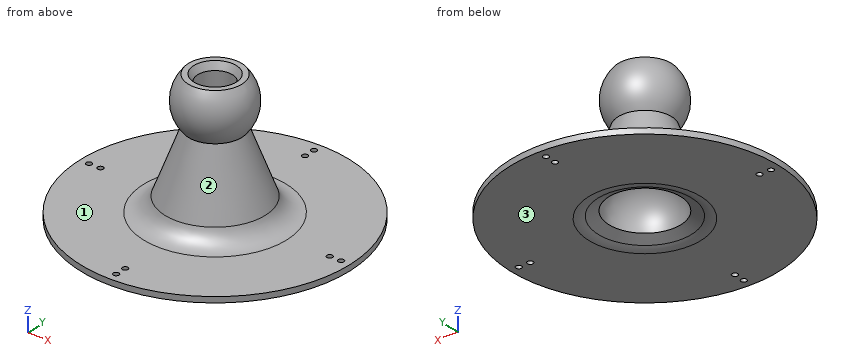
```python
from build123d import *

# Parameters (mm, degrees)
SKETCH2_R          = 28.533493352
CUT_EXTRUDE1_DEPTH = 3.900597164
CUT_EXTRUDE1_DRAFT = -65.378461827
HOLE1_D            = 3.175
HOLE1_DEPTH        = 72.381695866
CHAMFER1_SIZE      = 2.199704526
CHAMFER1_SIZE2     = 3.81
FILLET1_R          = 12.7


with BuildPart() as part:
    # Sketch1 → Revolve1 (revolve)
    with BuildSketch(Plane(origin=(0, 0, 0), x_dir=(1, 0, 0), z_dir=(0, 1, 0))):
        with BuildLine():
            Line((75, 1.293744634), (0, 1.293744634))
            Line((0, 1.293744634), (0, -2.606852529))
            Line((0, -2.606852529), (20.022304736, -2.606852529))
            ThreePointArc((20.022304736, -2.606852529), (17.926393777, -14.259573819), (9.652, -22.727936343))
            Line((9.652, -22.727936343), (9.652, -71.087951232))
            Line((9.652, -71.087951232), (14.88071719, -71.087951232))
            ThreePointArc((14.88071719, -71.087951232), (19.97075, -57.768975616), (14.88071719, -44.45))
            Line((14.88071719, -44.45), (31.064900574, -1.881255366))
            Line((31.064900574, -1.881255366), (75, -1.881255366))
            Line((75, -1.881255366), (75, 1.293744634))
        make_face()
    revolve(axis=Axis((0, 0, -1.293744634), (0, 0, 1)))


with BuildPart() as cut_extrude1_tool:
    # Sketch2 → Cut-Extrude1 (with draft: the straight prism first)
    with BuildSketch(Plane(origin=(0, 0, -1.293744634), x_dir=(-1, 0, 0), z_dir=(0, 0, -1))):
        Circle(SKETCH2_R)
    extrude(amount=-CUT_EXTRUDE1_DEPTH)
    # Cut-Extrude1: the draft: its side faces are tilted about the plane it starts from
    cut_extrude1_sides = [cut_extrude1_tool.faces().sort_by_distance(p)[0] for p in [
        (28.533493352, 0, 0.656553947),
    ]]
    draft(cut_extrude1_sides, Plane(origin=(0, 0, -1.293744634), x_dir=(-1, 0, 0), z_dir=(0, 0, -1)), CUT_EXTRUDE1_DRAFT)


with BuildPart() as part_1:
    add(part.part)

    # Cut-Extrude1: cut by cut_extrude1_tool
    add(cut_extrude1_tool.part, mode=Mode.SUBTRACT)

    # Hole1
    with Locations(Plane(origin=(0, 0, -1.293744634), x_dir=(-1, 0, 0), z_dir=(0, 0, -1))):
        with Locations((-63.5, 0), (-69.85, 0), (0, 63.5), (0, 69.85), (63.5, 0), (69.85, 0), (0, -63.5), (0, -69.85)):
            Hole(HOLE1_D / 2, depth=HOLE1_DEPTH)

    # Chamfer1
    chamfer1_edges = [part_1.edges().sort_by_distance(p)[0] for p in [
        (-9.652, 0, 71.087951232),
    ]]
    chamfer1_side = [part_1.faces().sort_by_distance(p)[0] for p in [
        (-10.072890241, 0, 71.087951232),
    ]]
    chamfer(chamfer1_edges, length=CHAMFER1_SIZE, length2=CHAMFER1_SIZE2, reference=chamfer1_side[0])

    # Fillet1
    fillet1_edges = [part_1.edges().sort_by_distance(p)[0] for p in [
        (-31.064900574, 0, 1.881255366),
        (28.533493352, 0, -1.293744634),
    ]]
    fillet(fillet1_edges, radius=FILLET1_R)


solid = part_1.part
```
The model under review builds one solid part; all positions refer to its coordinate system, in mm. Face numbers are marked on the shaded views. Round coordinates to 2 decimals unless told otherwise and drop trailing zeros. Order: outer loops, then holes, each group sorted by start corner. A loop starts at its lowest first (then second) coordinate and runs counter-clockwise, first axis right, second up. Notation, with made-up numbers: (2.5, -34.75) -> (25.5, -34.75) arc R11 ccw to (25.5, -17.75) -> close; hole circle Ø10 at (-39.75, 49.5). An arc over 180 degrees is marked (long way). Use a Markdown table: item, result.
Q1. Mouldability with a two-part tool opening along Z and no side actions: class the marked faces 1, 2 and 3 as +Z half, -Z half, draft (parallel to the pull), parting line (faces both ways), or undercut.
Values:
| item | result |
|---|---|
| face 1 | +Z half |
| face 2 | undercut |
| face 3 | -Z half |
Q2. We need section A-A on z = 33.5. Write out the cut boundary in (x, y), then the cut area to 3 significant figures.
Values:
| item | result |
|---|---|
| outline | circle Ø38.09 at (0, 0); hole circle Ø19.3 at (0, 0) |
| area | 847 mm^2 |
Q3. We need section B-B on x = 47. Write out the cut boundary in (y, z), then the cut area to 3 significant figures.
Values:
| item | result |
|---|---|
| outline | (-58.45, -1.29) -> (58.45, -1.29) -> (58.45, 1.88) -> (-58.45, 1.88) -> close |
| area | 371 mm^2 |
Q4. Clearance check with flat-ended pins moving along their axes: P1, Ø2.5, axis at x = 63.5, y = 0, coming from the +Z side; P2, Ø1, axis at x = -20, y = -15.5, coming from the -Z side; P3, Ø10, axis at x = 6.5, y = 20.5, coming from the -Z side; P4, Ø8, axis at x = -38, y = -50, coming from the +Z side. State where each tip first meets the part, or that it passes through.
Values:
| item | result |
|---|---|
| P1 | passes through |
| P2 | stops at z = -0.04 |
| P3 | stops at z = -0.35 |
| P4 | stops at z = 1.88 |
Q5. We need section C-C on y = 50. Write out the cut boundary in (x, z).
Values:
| item | result |
|---|---|
| outline | (-55.9, -1.29) -> (55.9, -1.29) -> (55.9, 1.88) -> (-55.9, 1.88) -> close |
Q6. For line 1 (Y direction, x = 0, z = 0.75); line 2 (Z direction, x = 46, y = -48); line 3 (Y direction, x = 0, z = 48), list the stretches that pass through material, from the lowest coordinate up.
Values:
| item | result |
|---|---|
| line 1 | y = -75 to -71.44, -68.26 to -65.09, -61.91 to -24.07, 24.07 to 61.91, 65.09 to 68.26, 71.44 to 75 |
| line 2 | z = -1.29 to 1.88 |
| line 3 | y = -17.42 to -9.65, 9.65 to 17.42 |
Q7. We need section D-D on z = 46.5. Write out the cut boundary in (x, y), then the cut area to 3 significant figures.
Values:
| item | result |
|---|---|
| outline | circle Ø32.98 at (0, 0); hole circle Ø19.3 at (0, 0) |
| area | 561 mm^2 |
